Verification items for the finished model (mm, model axes). A direction names the side the tool comes from. Give positions to 0.01 mm unless a question says otherwise; leave off trailing zeros. Loops run counter-clockwise (first coordinate to the right, second up) from the corner with the lowest first, then second, coordinate; pieces in that order, holes last. Notation, with made-up numbers: M 76.25,65 L 87.25,65 A7 ccw 87.25,71 Z; hole C -30,15.5 d7. An arc over 180 degrees is marked long. Write each question's results on one line, items separated by ' | '. Start each with the question number.
```python
from build123d import *

# Parameters (mm, degrees)
F0_W         = 500
F0_H         = 500
F1_DEPTH     = 10
F2_W         = 500
F2_H         = 10
F3_DEPTH     = 200
F4_W         = 10
F4_H         = 490
F5_DEPTH     = 250
F6_W         = 490
F6_H         = 10
F7_DEPTH     = 250
F8_W         = 10
F8_H         = 480
F9_DEPTH     = 250
F10_DEPTH    = 50
F10_FACE_W   = 500
F10_FACE_H   = 500
F10_FACE_W_2 = 480
F10_FACE_H_2 = 480
F11_DEPTH    = 50
F12_R        = 60
F13_DEPTH    = 70
F14_R        = 60
F15_DEPTH    = 122
F16_W        = 220
F16_H        = 45
F17_DEPTH    = 25
F18_R        = 60
F19_DEPTH    = 25
F20_R        = 60
F21_DEPTH    = 25


with BuildPart() as f1:
    # F0 (on Top) → F1 (new body)
    with BuildSketch(Plane.XY):
        with Locations((-198.410127, 219.103556)):
            Rectangle(F0_W, F0_H)
    extrude(amount=F1_DEPTH)

    # F2 (on face) → F3 (join)
    with BuildSketch(Plane.XY.offset(10)):
        with Locations((-198.410127, 464.103556)):
            Rectangle(F2_W, F2_H)
    extrude(amount=F3_DEPTH)

    # F4 (on face) → F5 (join)
    with BuildSketch(Plane.XY.offset(10)):
        with Locations((46.589873, 214.103556)):
            Rectangle(F4_W, F4_H)
    extrude(amount=F5_DEPTH)

    # F6 (on face) → F7 (join)
    with BuildSketch(Plane.XY.offset(10)):
        with Locations((-203.410127, -25.896444)):
            Rectangle(F6_W, F6_H)
    extrude(amount=F7_DEPTH)

    # F8 (on face) → F9 (join)
    with BuildSketch(Plane.XY.offset(10)):
        with Locations((-443.410127, 219.103556)):
            Rectangle(F8_W, F8_H)
    extrude(amount=F9_DEPTH)

    # F3_face (on face) → F10 (join)
    with BuildSketch(Plane(origin=(-198.410127, 464.103556, 210), x_dir=(1, 0, 0), z_dir=(0, 0, 1))):
        Polygon((-250, -5), (-240, -5), (240, -5), (250, -5), (250, 5), (-250, 5), align=None)
    extrude(amount=F10_DEPTH)

    # F10_face (on face) → F11 (cut)
    with BuildSketch(Plane(origin=(-198.410127, 219.103556, 260), x_dir=(1, 0, 0), z_dir=(0, 0, 1))):
        Rectangle(F10_FACE_W, F10_FACE_H)
        Rectangle(F10_FACE_W_2, F10_FACE_H_2, mode=Mode.SUBTRACT)
    extrude(amount=-F11_DEPTH, mode=Mode.SUBTRACT)

    # F12 (on face) → F13 (cut)
    with BuildSketch(Plane.XZ.offset(30.896444)):
        with Locations((-356.697887, 110.873759)):
            Circle(F12_R)
    extrude(amount=-F13_DEPTH, mode=Mode.SUBTRACT)

    # F14 (on face) → F15 (cut)
    with BuildSketch(Plane.XZ.offset(30.896444)):
        with Locations((-204.655066, 108.496942)):
            Circle(F14_R)
    extrude(amount=-F15_DEPTH, mode=Mode.SUBTRACT)

    # F16 (on face) → F17 (cut)
    with BuildSketch(Plane(origin=(-448.410127, 0, 0), x_dir=(0, -1, 0), z_dir=(-1, 0, 0))):
        with Locations((-89.816239, 39.089018)):
            Rectangle(F16_W, F16_H)
    extrude(amount=-F17_DEPTH, mode=Mode.SUBTRACT)

    # F18 (on face) → F19 (cut)
    with BuildSketch(Plane(origin=(-448.410127, 0, 0), x_dir=(0, -1, 0), z_dir=(-1, 0, 0))):
        with Locations((-393.093586, 107.814118)):
            Circle(F18_R)
    extrude(amount=-F19_DEPTH, mode=Mode.SUBTRACT)

    # F20 (on face) → F21 (cut)
    with BuildSketch(Plane(origin=(-448.410127, 0, 0), x_dir=(0, -1, 0), z_dir=(-1, 0, 0))):
        with Locations((-262.70619, 106.892653)):
            Circle(F20_R)
    extrude(amount=-F21_DEPTH, mode=Mode.SUBTRACT)


solid = f1.part
```
1. Section check B-B, the plane z = 76. Record the boundary of the cut face in (x, y).
2. Thickness scan on probe 1 along Y at (x, z) = (-97, 158.5); probe 2 along X at (y, z) = (60, 182); probe 3 along Y at (x, z) = (-239.5, 94.5). Record the ranges inside material, lowest first.
3. Section check A-A, the plane y = 170. Record the boundary of the cut face in (x, z), plus the area to 3 significant figures.
4. Release check for a two-part mould opening along Z. For faces 1 (the face through (-448.41, 167, 104)), 2 (the face through (-440, 331, 210)), 3 (the face through (-443.48, 322.65, 109.53)) record: released by +Z, released by -Z, zero draft, split by the parting line, or undercut.
5. Section check D-D, the plane x = -400. Record the boundary of the cut face in (y, z).
6. Section check C-C, the plane x = -32.5. Record the boundary of the cut face in (y, z), plus the area to 3 significant figures.
7. Depth check by flat-ended pin: pin 1 Ø11 at (x, y) = (-442, 66) entering from -Z; pin 2 Ø4 at (y, z) = (124.5, 45.5) entering from -X. Enter the tip coordinate at first touch or a pass-through.
8. Set-up check for faces 4 (the face through (-301.273, -25.966, 87.893)), 5 (the face through (-195, 469.104, 104)), 6 (the face through (-146, -30.896, 80)), 7 (the face through (-202, 459.104, 109)), 8 (the face through (-443.48, 406.1, 49.24)): record each of +Z, -Z, +X, -X, +Y, -Y from which the full face is reachable in a straight line by a thin tool's end or side.
Filled sheet:
1) outline: M -448.41,-30.9 L -405.52,-30.9 L -405.52,-20.9 L -438.41,-20.9 L -438.41,211.27 L -448.41,211.27 Z; M -448.41,314.14 L -438.41,314.14 L -438.41,342.22 L -448.41,342.22 Z; M -448.41,443.96 L -438.41,443.96 L -438.41,459.1 L 41.59,459.1 L 41.59,-20.9 L -154.22,-20.9 L -154.22,-30.9 L 51.59,-30.9 L 51.59,469.1 L -448.41,469.1 Z; M -307.87,-30.9 L -255.09,-30.9 L -255.09,-20.9 L -307.87,-20.9 Z
2) probe 1: -30.9 to -20.9, 459.1 to 469.1 | probe 2: -448.41 to -438.41, 41.59 to 51.59 | probe 3: 459.1 to 469.1
3) outline: M -448.41,0 L 51.59,0 L 51.59,210 L 41.59,210 L 41.59,10 L -438.41,10 L -438.41,16.59 L -448.41,16.59 Z; M -448.41,61.59 L -438.41,61.59 L -438.41,210 L -448.41,210 Z | area: 8,550 mm2
4) face 1: zero draft | face 2: released by +Z | face 3: undercut
5) outline: M -30.9,0 L 469.1,0 L 469.1,210 L 459.1,210 L 459.1,10 L -20.9,10 L -20.9,69.34 L -30.9,69.34 Z; M -30.9,152.41 L -20.9,152.41 L -20.9,210 L -30.9,210 Z
6) outline: M -30.9,0 L 469.1,0 L 469.1,210 L 459.1,210 L 459.1,10 L -20.9,10 L -20.9,210 L -30.9,210 Z | area: 9,000 mm2
7) pin 1: z = 0 | pin 2: x = 41.59
8) face 4: -Y | face 5: +Z, -Z, +X, -X, +Y | face 6: +Z, -Z, +X, -X, -Y | face 7: +Z | face 8: -X
